CAD build for the part. Positions are in the model's coordinates, mm. A direction names the side the tool comes from. Round coordinates to 2 decimals unless told otherwise and drop trailing zeros. Order: outer loops, then holes, each group sorted by start corner. A loop starts at its lowest first (then second) coordinate and runs counter-clockwise, first axis right, second up. Notation, with made-up numbers: (7.5, 34.5) - (63.5, 34.5) arc R30 cw to (63.5, 68.5) - close; hole circle Ø4 at (72.5, 67.5). An arc over 180 degrees is marked (long way). Write item = value, one per line.
from build123d import *

# Parameters (mm, degrees)
SKETCH1_R               = 27.5
BOSS_EXTRUDE1_DEPTH     = 1
SKETCH2_R               = 27.5
SKETCH2_R_2             = 16
BOSS_EXTRUDE2_DEPTH     = 8
SKETCH3_W               = 0.250349807
SKETCH3_H               = 12
BOSS_EXTRUDE3_DEPTH     = 60
CUT_EXTRUDE1_DEPTH      = 72.50174823
CUT_EXTRUDE1_DEPTH_BACK = 72.50174823
SKETCH4_R               = 2.5
SKETCH4_R_2             = 1
FILLET1_R               = 5


with BuildPart() as part:
    # Sketch1 → Boss-Extrude1 (new body)
    with BuildSketch(Plane.XY):
        Circle(SKETCH1_R)
    extrude(amount=BOSS_EXTRUDE1_DEPTH)

    # Sketch2 → Boss-Extrude2 (add)
    with BuildSketch(Plane.XY.offset(1)):
        Circle(SKETCH2_R)
        Circle(SKETCH2_R_2, mode=Mode.SUBTRACT)
    extrude(amount=BOSS_EXTRUDE2_DEPTH)

    # Sketch3 → Boss-Extrude3 (add)
    with BuildSketch(Plane(origin=(0, 0, 0), x_dir=(-1, 0, 0), z_dir=(0, 0, -1))):
        with Locations((-26.125174904, 0)):
            Rectangle(SKETCH3_W, SKETCH3_H)
        with Locations((26.125174904, 0)):
            Rectangle(SKETCH3_W, SKETCH3_H)
    extrude(amount=BOSS_EXTRUDE3_DEPTH)

    # Sketch4 → Cut-Extrude1 (cut, two sides: drawn at the far end of the back side and taken through both)
    with BuildSketch(Plane(origin=(0, 0, 0), x_dir=(0, 0, -1), z_dir=(1, 0, 0)).offset(-CUT_EXTRUDE1_DEPTH_BACK)):
        with Locations((37.113852525, 0)):
            Circle(SKETCH4_R)
        with Locations((4.573176496, 0)):
            Circle(SKETCH4_R_2)
    extrude(amount=CUT_EXTRUDE1_DEPTH + CUT_EXTRUDE1_DEPTH_BACK, mode=Mode.SUBTRACT)

    # Fillet1
    fillet1_edges = [part.edges().sort_by_distance(p)[0] for p in [
        (-26.125174903, -6, -60),
        (-26.125174903, 6, -60),
        (26.125174903, -6, -60),
        (26.125174903, 6, -60),
    ]]
    fillet(fillet1_edges, radius=FILLET1_R)


solid = part.part
(1) Tool access for faces 4 (the flat face through (26.25, 0, -30)), 5 (the flat face through (-26.25, 0, -30)), 6 (the flat face through (26, 0, -30)): list every direction of +Z, -Z, +X, -X, +Y, -Y with a clear straight run to the whole face (end or side of a thin tool).
Solved:
face_4 = -Z, +X, +Y, -Y
face_5 = -Z, -X, +Y, -Y
face_6 = -Z, +Y, -Y
(2) Drop flat-ended pins along their axis: pin 1 (1 mm diameter, centred on x = 13, y = -10, fed in from -Z); pin 2 (9.5 mm diameter, centred on x = -0.5, y = 1.5, fed in from +Z); pin 3 (6 mm diameter, centred on y = 0, z = -37.11, fed in from -X); pin 4 (1.2 mm diameter, centred on y = 0, z = -4.57, fed in from +X). Give the stop position or say it passes through.
Solved:
pin_1 = 0
pin_2 = 1
pin_3 = -26.25
pin_4 = through
(3) Probe line 1 along Z through (x, y) = (26.15, 0); line 2 along X through (y, z) = (-1, -31); line 3 along Z through (x, y) = (-20, 14). List the from-to ranges inside material, lowest first.
Solved:
line_1 = -60 to -39.61, -34.61 to -5.57, -3.57 to 9
line_2 = -26.25 to -26, 26 to 26.25
line_3 = 0 to 9
(4) Pull direction Y, two halves, no side cores. Call faces 1 (the flat face through (-26, 0, -30)), 2 (the flat face through (0, 0, 1)), 3 (the cylindrical face through (-5.961, -26.846, 4.437)): released by +Y, released by -Y, zero draft, split by the parting line, or undercut.
Solved:
face_1 = zero draft
face_2 = undercut
face_3 = split by the parting line
(5) Band-saw the part on B-B on z = -4.5. List the corners of the cut face in (x, y).
Solved:
outline = (-26.25, -6) - (-26, -6) - (-26, -1) - (-26.25, -1) - close; (-26.25, 1) - (-26, 1) - (-26, 6) - (-26.25, 6) - close; (26, -6) - (26.25, -6) - (26.25, -1) - (26, -1) - close; (26, 1) - (26.25, 1) - (26.25, 6) - (26, 6) - close
(6) Band-saw the part on D-D on z = -48.5. List the corners of the cut face in (x, y), plus the area to 3 significant figures.
Solved:
outline = (-26.25, -6) - (-26, -6) - (-26, 6) - (-26.25, 6) - close; (26, -6) - (26.25, -6) - (26.25, 6) - (26, 6) - close
area = 6.01 mm²
(7) Band-saw the part on A-A on y = 0. Count the separate pieces of the cut face and the enclosed holes in it, plus the area to 3 significant figures.
Solved:
separate_pieces = 5
enclosed_holes = 0
area = 266 mm²
(8) Band-saw the part on C-C on x = 0. List the corners of the cut face in (y, z).
Solved:
outline = (-27.5, 0) - (27.5, 0) - (27.5, 9) - (16, 9) - (16, 1) - (-16, 1) - (-16, 9) - (-27.5, 9) - close
